```python
from build123d import *

# Parameters (mm, degrees)
SKETCH1_W                = 16.2
SKETCH1_H                = 15.1
BOSS_EXTRUDE1_DEPTH      = 2.75
M1_CLEARANCE_HOLE2_D     = 1.2
M1_CLEARANCE_HOLE2_DEPTH = 2.75


with BuildPart() as part:
    # Sketch1 → Boss-Extrude1 (new body)
    with BuildSketch(Plane.XY):
        Rectangle(SKETCH1_W, SKETCH1_H)
    extrude(amount=BOSS_EXTRUDE1_DEPTH)

    # Sketch3 → M1 Clearance Hole1 (revolve, cut)
    with BuildSketch(Plane(origin=(7.1, 6.55, 2.75), x_dir=(0, -1, 0), z_dir=(1, 0, 0))):
        Polygon((0, 0), (0, 3.510516371), (0.6, 3.15), (0.6, 0), align=None)
    m1_clearance_hole1 = revolve(axis=Axis((7.1, 6.55, 9.1), (0, 0, -1)), mode=Mode.SUBTRACT)

    # Mirror1: M1 Clearance Hole1 across plane
    add(m1_clearance_hole1.mirror(Plane(origin=(0, 0, 0), x_dir=(0, 0, 1), z_dir=(1, 0, 0))), mode=Mode.SUBTRACT)

    # M1 Clearance Hole2
    with Locations(Plane.XY.offset(2.75)):
        with Locations((0, 6.55)):
            Hole(M1_CLEARANCE_HOLE2_D / 2, depth=M1_CLEARANCE_HOLE2_DEPTH)


solid = part.part
```
Build history of the part. All positions in model axes, mm. Give positions to 0.01 mm unless a question says otherwise; leave off trailing zeros. Loops run counter-clockwise (first coordinate to the right, second up) from the corner with the lowest first, then second, coordinate; pieces in that order, holes last. Notation, with made-up numbers: (-29, 50.5) - (12, 50.5) arc R23 cw to (12, 86.5) - close; hole circle Ø10 at (7, 77). An arc over 180 degrees is marked (long way). Use a Markdown table: item, result.
(1) Wall check: line 1 along Y through (x, z) = (7.1, 1.8); line 2 along X through (y, z) = (6.25, 2.15); line 3 along Y through (x, z) = (0.5, 1.25). Give the ranges that are in metal, low to high.
Taken from the geometry:
| item | result |
|---|---|
| line 1 | -7.55 to 5.95, 7.15 to 7.55 |
| line 2 | -8.1 to -7.62, -6.58 to -0.52, 0.52 to 6.58, 7.62 to 8.1 |
| line 3 | -7.55 to 6.22, 6.88 to 7.55 |
(2) Band-saw the part on A-A (x = 7.1). Give the cut face in (y, z).
Taken from the geometry:
| item | result |
|---|---|
| outline | (-7.55, 0) - (5.95, 0) - (5.95, 2.75) - (-7.55, 2.75) - close; (7.15, 0) - (7.55, 0) - (7.55, 2.75) - (7.15, 2.75) - close |
(3) Pull direction X, two halves, no side cores. Call faces 1 (the face through (0, 7.55, 1)), 2 (the face through (8.1, 0, 1)), 3 (the face through (-6.505, 6.628, 1.394)), 4 (the face through (6.505, 6.628, 1.394)): +X half, -X half, draft (parallel to the pull), parting line (faces both ways), or undercut.
Taken from the geometry:
| item | result |
|---|---|
| face 1 | draft |
| face 2 | +X half |
| face 3 | undercut |
| face 4 | undercut |
(4) Drop flat-ended pins along their axis: pin 1 Ø5 at (x, y) = (-1, -6) entering from -Z; pin 2 Ø0.7 at (x, y) = (0, 6.55) entering from -Z. Give the stop position or say it passes through.
Taken from the geometry:
| item | result |
|---|---|
| pin 1 | z = 0 |
| pin 2 | through |
(5) Band-saw the part on B-B (y = 6.55). Give the cut face in (x, z), and give its area (4 significant figures).
Taken from the geometry:
| item | result |
|---|---|
| outline | (-8.1, 0) - (-7.7, 0) - (-7.7, 2.75) - (-8.1, 2.75) - close; (-6.5, 0) - (-0.6, 0) - (-0.6, 2.75) - (-6.5, 2.75) - close; (0.6, 0) - (6.5, 0) - (6.5, 2.75) - (0.6, 2.75) - close; (7.7, 0) - (8.1, 0) - (8.1, 2.75) - (7.7, 2.75) - close |
| area | 34.65 mm2 |
